```python
from build123d import *

# Parameters (mm, degrees)
DODANIE_WYCI_GNI_CIE1_DEPTH            = 7
WYTNIJ_WYCI_GNI_CIE1_REACH             = 28.495
WYTNIJ_WYCI_GNI_CIE2_REACH             = 28.495
SZKIC3_R                               = 1.5
SZKIC4_W                               = 22
SZKIC4_H                               = 17
DODANIE_WYCI_GNI_CIE2_DEPTH            = 20
SZKIC5_R                               = 3
WYTNIJ_WYCI_GNI_CIE3_DEPTH             = 20
WYTNIJ_WYCI_GNI_CIE4_DEPTH             = 2.5
WYTNIJ_WYCI_GNI_CIE5_REACH             = 30.46
SZKIC7_R                               = 1.5
WYTNIJ_WYCI_GNI_CIE5_DIRECTION_2_REACH = 30.46
DODANIE_WYCI_GNI_CIE3_START            = 15
SZKIC8_W                               = 9
SZKIC8_H                               = 17
SZKIC8_R                               = 3
DODANIE_WYCI_GNI_CIE3_DEPTH            = 15
SZKIC9_R                               = 1.5
WYTNIJ_WYCI_GNI_CIE6_DEPTH             = 9


with BuildPart() as part:
    # Szkic1 → Dodanie-wyciągnięcie1 (new body)
    with BuildSketch(Plane.XY):
        Polygon((8, 6), (-8, 6), (-11, 6), (-11, -13), (-8, -13), (-8, -6), (8, -6), (8, -13), (11, -13), (11, 6), align=None)
    extrude(amount=DODANIE_WYCI_GNI_CIE1_DEPTH)

    # Wytnij-wyciągnięcie1: up to this face of the body (flat: up to its plane)
    wytnij_wyci_gni_cie1_end = Plane(part.part.faces().sort_by_distance((11, -3.5, 3.5))[0])
    # Szkic2 → Wytnij-wyciągnięcie1 (cut, up to the picked face)
    with BuildSketch(Plane.ZY.offset(11), mode=Mode.PRIVATE) as wytnij_wyci_gni_cie1_sk1:
        with BuildLine():
            ThreePointArc((7, -9.5), (5.974873734, -11.974873734), (3.5, -13))
            Line((3.5, -13), (7, -13))
            Line((7, -13), (7, -9.5))
        make_face()
    wytnij_wyci_gni_cie1_tool1 = split(extrude(wytnij_wyci_gni_cie1_sk1.sketch, amount=-WYTNIJ_WYCI_GNI_CIE1_REACH, mode=Mode.PRIVATE), bisect_by=wytnij_wyci_gni_cie1_end, keep=Keep.BOTH, mode=Mode.PRIVATE)
    # Szkic2 → Wytnij-wyciągnięcie1 (cut, up to the picked face)
    with BuildSketch(Plane.ZY.offset(11), mode=Mode.PRIVATE) as wytnij_wyci_gni_cie1_sk2:
        with BuildLine():
            ThreePointArc((3.5, -13), (1.025126266, -11.974873734), (0, -9.5))
            Line((0, -9.5), (0, -13))
            Line((0, -13), (3.5, -13))
        make_face()
    wytnij_wyci_gni_cie1_tool2 = split(extrude(wytnij_wyci_gni_cie1_sk2.sketch, amount=-WYTNIJ_WYCI_GNI_CIE1_REACH, mode=Mode.PRIVATE), bisect_by=wytnij_wyci_gni_cie1_end, keep=Keep.BOTH, mode=Mode.PRIVATE)
    add(wytnij_wyci_gni_cie1_tool1.solids().sort_by(Axis((-11, -12.218212, 6.218212), (1, 0, 0)))[0], mode=Mode.SUBTRACT)
    add(wytnij_wyci_gni_cie1_tool2.solids().sort_by(Axis((-11, -12.218212, 0.781788), (1, 0, 0)))[0], mode=Mode.SUBTRACT)

    # Wytnij-wyciągnięcie2: up to this face of the body (flat: up to its plane)
    wytnij_wyci_gni_cie2_end = Plane(part.part.faces().sort_by_distance((11, -3.141167, 3.5))[0])
    # Szkic3 → Wytnij-wyciągnięcie2 (cut, up to the picked face)
    with BuildSketch(Plane.ZY.offset(11), mode=Mode.PRIVATE) as wytnij_wyci_gni_cie2_sk1:
        with Locations(Location((3.5, -10, 0), (0, 0, 270))):
            Circle(SZKIC3_R)
    wytnij_wyci_gni_cie2_tool1 = split(extrude(wytnij_wyci_gni_cie2_sk1.sketch, amount=-WYTNIJ_WYCI_GNI_CIE2_REACH, mode=Mode.PRIVATE), bisect_by=wytnij_wyci_gni_cie2_end, keep=Keep.BOTH, mode=Mode.PRIVATE)
    add(wytnij_wyci_gni_cie2_tool1.solids().sort_by(Axis((-11, -10, 3.5), (1, 0, 0)))[0], mode=Mode.SUBTRACT)

    # Szkic4 → Dodanie-wyciągnięcie2 (add)
    with BuildSketch(Plane(origin=(0, 0, 0), x_dir=(-1, 0, 0), z_dir=(0, 0, -1))):
        with Locations((0, 2.5)):
            Rectangle(SZKIC4_W, SZKIC4_H)
    extrude(amount=-DODANIE_WYCI_GNI_CIE2_DEPTH)

    # Szkic5 → Wytnij-wyciągnięcie3 (cut)
    with BuildSketch(Plane.XY.offset(20)):
        Circle(SZKIC5_R)
    extrude(amount=-WYTNIJ_WYCI_GNI_CIE3_DEPTH, mode=Mode.SUBTRACT)

    # Szkic6 → Wytnij-wyciągnięcie4 (cut)
    with BuildSketch(Plane(origin=(0, 4, 0), x_dir=(-1, 0, 0), z_dir=(0, -1, 0))):
        Polygon((2.65, -2.316843521), (2.65, 0), (-2.65, 0), (-2.65, -2.316843521), (-2.65, -5.376799948), (0, -6.906778161), (2.65, -5.376799948), align=None)
    extrude(amount=-WYTNIJ_WYCI_GNI_CIE4_DEPTH, mode=Mode.SUBTRACT)

    # Szkic7 → Wytnij-wyciągnięcie5 (cut, up to next)
    with BuildSketch(Plane(origin=(0, 4, 0), x_dir=(1, 0, 0), z_dir=(0, 1, 0)), mode=Mode.PRIVATE) as wytnij_wyci_gni_cie5_sk1:
        with Locations(Location((0, -4, 0), (0, 0, 270))):
            Circle(SZKIC7_R)
    wytnij_wyci_gni_cie5_tool1 = extrude(wytnij_wyci_gni_cie5_sk1.sketch, amount=-WYTNIJ_WYCI_GNI_CIE5_REACH, mode=Mode.PRIVATE) & part.part
    add(wytnij_wyci_gni_cie5_tool1.solids().sort_by_distance((0, 4, 4))[0], mode=Mode.SUBTRACT)

    # Szkic7 → Wytnij-wyciągnięcie5 direction 2 (cut, up to next)
    with BuildSketch(Plane(origin=(0, 4, 0), x_dir=(1, 0, 0), z_dir=(0, 1, 0)), mode=Mode.PRIVATE) as wytnij_wyci_gni_cie5_direction_2_sk1:
        with Locations(Location((0, -4, 0), (0, 0, 270))):
            Circle(SZKIC7_R)
    wytnij_wyci_gni_cie5_direction_2_tool1 = extrude(wytnij_wyci_gni_cie5_direction_2_sk1.sketch, amount=WYTNIJ_WYCI_GNI_CIE5_DIRECTION_2_REACH, mode=Mode.PRIVATE) & part.part
    add(wytnij_wyci_gni_cie5_direction_2_tool1.solids().sort_by_distance((0, 4, 4))[0], mode=Mode.SUBTRACT)

    # Szkic8 → Dodanie-wyciągnięcie3 (add)
    with BuildSketch(Plane.XY.offset(20).offset(DODANIE_WYCI_GNI_CIE3_START)):
        with Locations((0, 2.5)):
            Rectangle(SZKIC8_W, SZKIC8_H)
        Circle(SZKIC8_R, mode=Mode.SUBTRACT)
    extrude(amount=-DODANIE_WYCI_GNI_CIE3_DEPTH)

    # Szkic9 → Wytnij-wyciągnięcie6 (cut)
    with BuildSketch(Plane(origin=(4.5, 0, 0), x_dir=(0, 0, -1), z_dir=(1, 0, 0))):
        with Locations(Location((-31, 8, 0), (0, 0, 90))):
            Circle(SZKIC9_R)
    extrude(amount=-WYTNIJ_WYCI_GNI_CIE6_DEPTH, mode=Mode.SUBTRACT)


solid = part.part
```
For this review, take the finished solid that the model builds, in its own axes (mm). A direction names the side the tool comes from. Coordinates: 2 decimals unless noted, no trailing zeros. Order: outer loops, then holes, each group sorted by start corner. A loop starts at its lowest first (then second) coordinate and runs counter-clockwise, first axis right, second up. Notation, with made-up numbers: (39.25, 31) - (92.25, 31) arc R26 cw to (92.25, 63) - close; hole circle Ø11 at (62.25, 79). An arc over 180 degrees is marked (long way). Answer as a JSON object with one key per item and string values. Group by question number.
1. Clearance check with flat-ended pins moving along their axes: P1, Ø1, axis at x = -5.5, z = 23, coming from the -Y side; P2, Ø2.5, axis at x = 1, z = 3.5, coming from the -Y side; P3, Ø1, axis at x = 0.5, z = 4.5, coming from the +Y side; P4, Ø1.8, axis at x = 0, z = 4, coming from the +Y side. State where each tip first meets the part, or that it passes through.
2. We need section D-D on y = 0. State the section outline as (x, z) points.
3. For probe 1 along Y at (x, z) = (-1.75, 4); probe 2 along X at (y, z) = (2.95, 4); probe 3 along Z at (x, y) = (-0.5, 9), list the stretches that pass through material, from the lowest coordinate up.
4. We need section B-B on z = 31. State the section outline as (x, y) points.
5. We need section C-C on x = 4. State the section outline as (y, z) points, then the cut area to 3 significant figures.
6. The part is to be moulded in two halves that separate along Z. For faces 1 (the flat face through (0, 5, 35)), 2 (the cylindrical face through (-9.5, -8.8, 2.6)), 3 (the flat face through (-2.65, 5, 3)), say which applies: pulls with the +Z half, pulls with the -Z half, needs draft (parallel to the pull), parting line crosses it, or undercut.
7. For faces 4 (the flat face through (-8, 3, 20)), 5 (the flat face through (1.344, 5.232, 6.131)), 6 (the flat face through (-10, -8, 7)), list the 3-axis set-ups (+Z, -Z, +X, -X, +Y, -Y) from which the entire face can be reached by the end or side of a thin tool; tool diameter is ignored.
8. We need section A-A on y = 8. State the section outline as (x, z) points.
Final values:
{
 "1": {"P1": "through", "P2": "y = -6", "P3": "y = -2.83", "P4": "y = -2.86"},
 "2": {"outline": "(-11, 0) - (-3, 0) - (-3, 35) - (-4.5, 35) - (-4.5, 20) - (-11, 20) - close; (3, 0) - (11, 0) - (11, 20) - (4.5, 20) - (4.5, 35) - (3, 35) - close"},
 "3": {"probe 1": "-6 to -2.44, 2.44 to 4, 6.5 to 11", "probe 2": "-11 to -1.5, 1.5 to 11", "probe 3": "0 to 2.59, 5.41 to 29.88, 32.12 to 35"},
 "4": {"outline": "(-4.5, -6) - (4.5, -6) - (4.5, 6.5) - (-4.5, 6.5) - close; (-4.5, 9.5) - (4.5, 9.5) - (4.5, 11) - (-4.5, 11) - close; hole circle Ø6 at (0, 0)"},
 "5": {"outline": "(-6, 0) - (11, 0) - (11, 35) - (-6, 35) - close; hole circle Ø3 at (8, 31)", "area": "588 mm²"},
 "6": {"face 1": "pulls with the +Z half", "face 2": "undercut", "face 3": "needs draft"},
 "7": {"face 4": "+Z, -X, +Y, -Y", "face 5": "-Z", "face 6": "+Z, +X, -X, -Y"},
 "8": {"outline": "(-11, 0) - (11, 0) - (11, 20) - (4.5, 20) - (4.5, 29.5) - (-4.5, 29.5) - (-4.5, 20) - (-11, 20) - close; (-4.5, 32.5) - (4.5, 32.5) - (4.5, 35) - (-4.5, 35) - close; hole circle Ø3 at (0, 4)"}
}
